Here's the drawing with two shaded views (mm, measured from the low corner). I have some questions. Give positions to 0.01 mm unless a question says otherwise; leave off trailing zeros. Write each loop counter-clockwise with the first axis right and the second up, starting at its lowest first coordinate (ties: lowest second). Pieces come first, ordered by that corner, then holes. Notation, with made-up numbers: (78, 9) - (90, 9) arc R18 cw to (90, 17) - close; hole circle Ø5 at (32.25, 84). An arc over 180 degrees is marked (long way). Use one line per item in the form item = value.
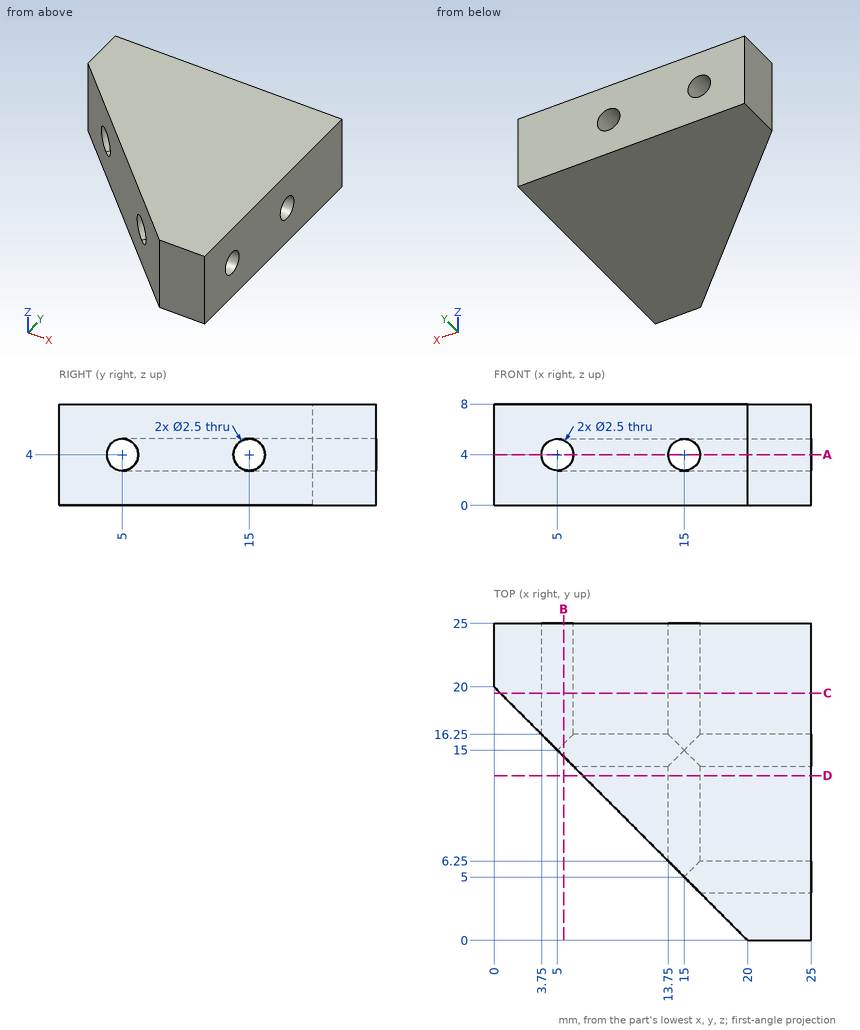
1. For pin 1 (4 mm diameter, centred on x = 11.5, z = 1, fed in from -Y); pin 2 (3 mm diameter, centred on y = 5, z = 4, fed in from -X), each with a flat end and sliding along its axis, tell me the tip position at first contact or that it passes through.
Response values:
pin_1 = 6.5
pin_2 = 13.5
2. Imagine slicing it at D-D, the plane y = 13. List the corners of the cut face in (x, z) for me.
Response values:
outline = (7, 0) - (25, 0) - (25, 8) - (7, 8) - close; hole circle Ø2.5 at (15, 4)
3. Imagine slicing it at B-B, the plane x = 5.5. List the corners of the cut face in (y, z) for me, and give its area (3 significant figures).
Response values:
outline = (14.5, 0) - (25, 0) - (25, 2.85) - (15.5, 2.85) arc R1.25 cw to (14.5, 2.85) - close; (14.5, 5.15) arc R1.25 cw to (15.5, 5.15) - (25, 5.15) - (25, 8) - (14.5, 8) - close
area = 59.8 mm²
4. If I drill on line 1 (Y direction, x = 20.25, z = 4); line 2 (Z direction, x = 15, y = 12.75), over which ranges is the centre line in solid material (lowest first)? Write a range as from..to.
Response values:
line_1 = 0..3.75, 6.25..13.75, 16.25..25
line_2 = 0..2.75, 5.25..8
5. Imagine slicing it at C-C, the plane y = 19.5. List the corners of the cut face in (x, z) for me.
Response values:
outline = (0.5, 0) - (25, 0) - (25, 8) - (0.5, 8) - close; hole circle Ø2.5 at (5, 4); hole circle Ø2.5 at (15, 4)
6. Imagine slicing it at A-A, the plane z = 4. List the corners of the cut face in (x, y) for me, and give its area (4 significant figures).
Response values:
outline = (0, 20) - (3.75, 16.25) - (3.75, 25) - (0, 25) - close; (6.25, 13.75) - (13.75, 6.25) - (13.75, 13.75) - close; (6.25, 16.25) - (13.75, 16.25) - (13.75, 25) - (6.25, 25) - close; (16.25, 3.75) - (20, 0) - (25, 0) - (25, 3.75) - close; (16.25, 6.25) - (25, 6.25) - (25, 13.75) - (16.25, 13.75) - close; (16.25, 16.25) - (25, 16.25) - (25, 25) - (16.25, 25) - close
area = 287.5 mm²
